Model file for the job. Use its own axes, mm. A direction names the side the tool comes from. Give positions to 0.01 mm unless a question says otherwise; leave off trailing zeros. Loops run counter-clockwise (first coordinate to the right, second up) from the corner with the lowest first, then second, coordinate; pieces in that order, holes last. Notation, with made-up numbers: M 35,47.25 L 65,47.25 A28 cw 65,75.25 Z; hole C 42,25.5 d8. An arc over 180 degrees is marked long. Answer in a Markdown table with one row per item.
```python
from build123d import *

# Parameters (mm, degrees)
BOSS_EXTRUDE1_DEPTH = 3
SKETCH2_R           = 1.6
CUT_EXTRUDE1_DEPTH  = 3


with BuildPart() as part:
    # Sketch1 → Boss-Extrude1 (new body)
    with BuildSketch(Plane.XY):
        with BuildLine():
            Line((-1.5, -3.16227766), (-1.5, 0))
            Line((-1.5, 0), (1.5, 0))
            Line((1.5, 0), (1.5, -3.16227766))
            ThreePointArc((1.5, -3.16227766), (2.958039892, -1.870828693), (3.5, 0))
            ThreePointArc((3.5, 0), (-1.870828693, 2.958039892), (-1.5, -3.16227766))
        make_face()
        with BuildLine():
            Line((1.5, 0), (-1.5, 0))
            Line((-1.5, 0), (-1.5, -3.16227766))
            ThreePointArc((-1.5, -3.16227766), (0, -3.5), (1.5, -3.16227766))
            Line((1.5, -3.16227766), (1.5, 0))
        make_face()
        with BuildLine():
            ThreePointArc((1.5, -3.16227766), (0, -3.5), (-1.5, -3.16227766))
            Line((-1.5, -3.16227766), (-1.5, -16.83772234))
            ThreePointArc((-1.5, -16.83772234), (0, -16.5), (1.5, -16.83772234))
            Line((1.5, -16.83772234), (1.5, -3.16227766))
        make_face()
        with BuildLine():
            ThreePointArc((1.5, -16.83772234), (0, -16.5), (-1.5, -16.83772234))
            Line((-1.5, -16.83772234), (-1.5, -20))
            Line((-1.5, -20), (1.5, -20))
            Line((1.5, -20), (1.5, -16.83772234))
        make_face()
        with BuildLine():
            Line((-1.5, -20), (-1.5, -16.83772234))
            ThreePointArc((-1.5, -16.83772234), (-1.870828693, -22.958039892), (3.5, -20))
            ThreePointArc((3.5, -20), (2.958039892, -18.129171307), (1.5, -16.83772234))
            Line((1.5, -16.83772234), (1.5, -20))
            Line((1.5, -20), (-1.5, -20))
        make_face()
    extrude(amount=BOSS_EXTRUDE1_DEPTH)

    # Sketch2 → Cut-Extrude1 (cut)
    with BuildSketch(Plane.XY.offset(3)):
        with Locations((0, -20)):
            Circle(SKETCH2_R)
        Circle(SKETCH2_R)
    extrude(amount=-CUT_EXTRUDE1_DEPTH, mode=Mode.SUBTRACT)


solid = part.part
```
Q1. Saw through at D-D (x = -2.5). Give the cut face in (y, z).
Reported:
| item | result |
|---|---|
| outline | M -22.45,0 L -17.55,0 L -17.55,3 L -22.45,3 Z; M -2.45,0 L 2.45,0 L 2.45,3 L -2.45,3 Z |
Q2. Saw through at B-B (z = 0.6). Give the cut face in (x, y), and give its area (3 significant figures).
Reported:
| item | result |
|---|---|
| outline | M -1.5,-16.84 A3.5 ccw long 1.5,-16.84 L 1.5,-3.16 A3.5 ccw long -1.5,-3.16 Z; hole C 0,-20 d3.2; hole C 0,0 d3.2 |
| area | 101 mm² |
Q3. Drop flat-ended pins along their axis: pin 1 (3 mm diameter, centred on x = 0, y = -20, fed in from +Z); pin 2 (0.9 mm diameter, centred on y = -8.5, z = 2, fed in from +X). Give the stop position or say it passes through.
Reported:
| item | result |
|---|---|
| pin 1 | through |
| pin 2 | x = 1.5 |
Q4. 3-axis set-ups, long thin cutter, end or side, ignore diameter. For faces 1 (the face through (0, -10, 0)), 2 (the face through (-1.5, -10, 1)): which of +Z, -Z, +X, -X, +Y, -Y reach the whole face in a straight line?
Reported:
| item | result |
|---|---|
| face 1 | -Z, +X, -X, +Y, -Y |
| face 2 | +Z, -Z, -X |
Q5. Saw through at A-A (x = 0). Give the cut face in (y, z).
Reported:
| item | result |
|---|---|
| outline | M -23.5,0 L -21.6,0 L -21.6,3 L -23.5,3 Z; M -18.4,0 L -1.6,0 L -1.6,3 L -18.4,3 Z; M 1.6,0 L 3.5,0 L 3.5,3 L 1.6,3 Z |
Q6. Mould opens along Y. For faces 3 (the face through (1.5, -10, 1)), 4 (the face through (0, -10, 3)) say: released by +Y, released by -Y, zero draft, split by the parting line, or undercut.
Reported:
| item | result |
|---|---|
| face 3 | undercut |
| face 4 | zero draft |
Q7. Probe probe 1 along Y at (x, z) = (0, 1.05); probe 2 along Y at (x, z) = (0.5, 2.35); probe 3 along X at (y, z) = (-9.5, 2.75). List the from-to ranges inside material, lowest first.
Reported:
| item | result |
|---|---|
| probe 1 | -23.5 to -21.6, -18.4 to -1.6, 1.6 to 3.5 |
| probe 2 | -23.46 to -21.52, -18.48 to -1.52, 1.52 to 3.46 |
| probe 3 | -1.5 to 1.5 |
Q8. Saw through at C-C (y = -0.5). Give the cut face in (x, z), and give its area (3 significant figures).
Reported:
| item | result |
|---|---|
| outline | M -3.46,0 L -1.52,0 L -1.52,3 L -3.46,3 Z; M 1.52,0 L 3.46,0 L 3.46,3 L 1.52,3 Z |
| area | 11.7 mm² |
